The model under review builds one solid part; all positions refer to its coordinate system, in mm. A direction names the side the tool comes from. Round coordinates to 2 decimals unless told otherwise and drop trailing zeros. Loops run counter-clockwise (first coordinate to the right, second up) from the corner with the lowest first, then second, coordinate; pieces in that order, holes last. Notation, with made-up numbers: M -4.5,-8.75 L 52.5,-8.75 A18 cw 52.5,19.25 Z; hole C 87,-15 d11. An arc over 180 degrees is marked long. One line per question, with ' | ' between items.
from build123d import *

# Parameters (mm, degrees)
SKETCH1_R           = 50
BOSS_EXTRUDE1_DEPTH = 5
SKETCH2_R           = 7
BOSS_EXTRUDE2_DEPTH = 2
CUT_EXTRUDE1_REACH  = 7
SKETCH3_R           = 1.55


with BuildPart() as part:
    # Sketch1 → Boss-Extrude1 (new body)
    with BuildSketch(Plane.XY):
        Circle(SKETCH1_R)
        with BuildLine():
            ThreePointArc((-31.028947368, -9.767518887), (-28.10136985, -6.783592054), (-26.375, -2.976470225))
            Line((-26.375, -2.976470225), (-26.375, 2.976470225))
            ThreePointArc((-26.375, 2.976470225), (-28.10136985, 6.783592054), (-31.028947368, 9.767518887))
            ThreePointArc((-31.028947368, 9.767518887), (-34.223647748, 14.6974406), (-33.189728353, 20.480281537))
            ThreePointArc((-33.189728353, 20.480281537), (-27.577164466, 27.577164466), (-20.480281537, 33.189728353))
            ThreePointArc((-20.480281537, 33.189728353), (-14.6974406, 34.223647748), (-9.767518887, 31.028947368))
            ThreePointArc((-9.767518887, 31.028947368), (0, 26), (9.767518887, 31.028947368))
            ThreePointArc((9.767518887, 31.028947368), (14.6974406, 34.223647748), (20.480281537, 33.189728353))
            ThreePointArc((20.480281537, 33.189728353), (27.577164466, 27.577164466), (33.189728353, 20.480281537))
            ThreePointArc((33.189728353, 20.480281537), (34.223647748, 14.6974406), (31.028947368, 9.767518887))
            ThreePointArc((31.028947368, 9.767518887), (28.10136985, 6.783592054), (26.375, 2.976470225))
            Line((26.375, 2.976470225), (26.375, -2.976470225))
            ThreePointArc((26.375, -2.976470225), (28.10136985, -6.783592054), (31.028947368, -9.767518887))
            ThreePointArc((31.028947368, -9.767518887), (34.223647748, -14.6974406), (33.189728353, -20.480281537))
            ThreePointArc((33.189728353, -20.480281537), (27.577164466, -27.577164466), (20.480281537, -33.189728353))
            ThreePointArc((20.480281537, -33.189728353), (14.6974406, -34.223647748), (9.767518887, -31.028947368))
            ThreePointArc((9.767518887, -31.028947368), (0, -26), (-9.767518887, -31.028947368))
            ThreePointArc((-9.767518887, -31.028947368), (-14.6974406, -34.223647748), (-20.480281537, -33.189728353))
            ThreePointArc((-20.480281537, -33.189728353), (-27.577164466, -27.577164466), (-33.189728353, -20.480281537))
            ThreePointArc((-33.189728353, -20.480281537), (-34.223647748, -14.6974406), (-31.028947368, -9.767518887))
        make_face(mode=Mode.SUBTRACT)
    extrude(amount=BOSS_EXTRUDE1_DEPTH)

    # Sketch2 → Boss-Extrude2 (add)
    with BuildSketch(Plane.XY.offset(5)):
        with Locations((-38, 0)):
            Circle(SKETCH2_R)
        with Locations((0, 38)):
            Circle(SKETCH2_R)
        with Locations((38, 0)):
            Circle(SKETCH2_R)
        with Locations((0, -38)):
            Circle(SKETCH2_R)
    extrude(amount=BOSS_EXTRUDE2_DEPTH)

    # Sketch3 → Cut-Extrude1 (cut, up to next)
    with BuildSketch(Plane.XY.offset(5), mode=Mode.PRIVATE) as cut_extrude1_sk1:
        with Locations((-12.727922061, 38.183766184)):
            Circle(SKETCH3_R)
    cut_extrude1_tool1 = extrude(cut_extrude1_sk1.sketch, amount=-CUT_EXTRUDE1_REACH, mode=Mode.PRIVATE) & part.part
    add(cut_extrude1_tool1.solids().sort_by_distance((-12.727922, 38.183766, 5))[0], mode=Mode.SUBTRACT)
    # Sketch3 → Cut-Extrude1 (cut, up to next)
    with BuildSketch(Plane.XY.offset(5), mode=Mode.PRIVATE) as cut_extrude1_sk2:
        with Locations((38.183766184, 12.727922061)):
            Circle(SKETCH3_R)
    cut_extrude1_tool2 = extrude(cut_extrude1_sk2.sketch, amount=-CUT_EXTRUDE1_REACH, mode=Mode.PRIVATE) & part.part
    add(cut_extrude1_tool2.solids().sort_by_distance((38.183766, 12.727922, 5))[0], mode=Mode.SUBTRACT)
    # Sketch3 → Cut-Extrude1 (cut, up to next)
    with BuildSketch(Plane.XY.offset(5), mode=Mode.PRIVATE) as cut_extrude1_sk3:
        with Locations((12.727922061, -38.183766184)):
            Circle(SKETCH3_R)
    cut_extrude1_tool3 = extrude(cut_extrude1_sk3.sketch, amount=-CUT_EXTRUDE1_REACH, mode=Mode.PRIVATE) & part.part
    add(cut_extrude1_tool3.solids().sort_by_distance((12.727922, -38.183766, 5))[0], mode=Mode.SUBTRACT)
    # Sketch3 → Cut-Extrude1 (cut, up to next)
    with BuildSketch(Plane.XY.offset(5), mode=Mode.PRIVATE) as cut_extrude1_sk4:
        with Locations((-38.183766184, -12.727922061)):
            Circle(SKETCH3_R)
    cut_extrude1_tool4 = extrude(cut_extrude1_sk4.sketch, amount=-CUT_EXTRUDE1_REACH, mode=Mode.PRIVATE) & part.part
    add(cut_extrude1_tool4.solids().sort_by_distance((-38.183766, -12.727922, 5))[0], mode=Mode.SUBTRACT)
    # Sketch3 → Cut-Extrude1 (cut, up to next)
    with BuildSketch(Plane.XY.offset(5), mode=Mode.PRIVATE) as cut_extrude1_sk5:
        with Locations((-38.183766184, 12.727922061)):
            Circle(SKETCH3_R)
    cut_extrude1_tool5 = extrude(cut_extrude1_sk5.sketch, amount=-CUT_EXTRUDE1_REACH, mode=Mode.PRIVATE) & part.part
    add(cut_extrude1_tool5.solids().sort_by_distance((-38.183766, 12.727922, 5))[0], mode=Mode.SUBTRACT)
    # Sketch3 → Cut-Extrude1 (cut, up to next)
    with BuildSketch(Plane.XY.offset(5), mode=Mode.PRIVATE) as cut_extrude1_sk6:
        with Locations((12.727922061, 38.183766184)):
            Circle(SKETCH3_R)
    cut_extrude1_tool6 = extrude(cut_extrude1_sk6.sketch, amount=-CUT_EXTRUDE1_REACH, mode=Mode.PRIVATE) & part.part
    add(cut_extrude1_tool6.solids().sort_by_distance((12.727922, 38.183766, 5))[0], mode=Mode.SUBTRACT)
    # Sketch3 → Cut-Extrude1 (cut, up to next)
    with BuildSketch(Plane.XY.offset(5), mode=Mode.PRIVATE) as cut_extrude1_sk7:
        with Locations((38.183766184, -12.727922061)):
            Circle(SKETCH3_R)
    cut_extrude1_tool7 = extrude(cut_extrude1_sk7.sketch, amount=-CUT_EXTRUDE1_REACH, mode=Mode.PRIVATE) & part.part
    add(cut_extrude1_tool7.solids().sort_by_distance((38.183766, -12.727922, 5))[0], mode=Mode.SUBTRACT)
    # Sketch3 → Cut-Extrude1 (cut, up to next)
    with BuildSketch(Plane.XY.offset(5), mode=Mode.PRIVATE) as cut_extrude1_sk8:
        with Locations((-12.727922061, -38.183766184)):
            Circle(SKETCH3_R)
    cut_extrude1_tool8 = extrude(cut_extrude1_sk8.sketch, amount=-CUT_EXTRUDE1_REACH, mode=Mode.PRIVATE) & part.part
    add(cut_extrude1_tool8.solids().sort_by_distance((-12.727922, -38.183766, 5))[0], mode=Mode.SUBTRACT)


solid = part.part
1) Machinability: for faces 4 (the cylindrical face through (0, 26, 2)), 5 (the cylindrical face through (-0.91, -31.06, 5.99)), which of the approach directions +Z, -Z, +X, -X, +Y, -Y give a long, thin tool a straight path to every point of the face, cutting with its end or side? Answer none if there is none.
Output values:
face 4: +Z, -Z | face 5: +Z
2) Mouldability with a two-part tool opening along Y and no side actions: class faces 1 (the flat face through (0, 38, 7)), 2 (the cylindrical face through (44.677, 2.103, 5.986)), 3 (the cylindrical face through (14.615, 34.207, 2.465)) as +Y half, -Y half, draft (parallel to the pull), parting line (faces both ways), or undercut.
Output values:
face 1: draft | face 2: parting line | face 3: undercut
3) Add section C-C on x = -38. State the section outline as (y, z) points.
Output values:
outline: M -32.5,0 L -14.27,0 L -14.27,5 L -32.5,5 Z; M -11.19,0 L 11.19,0 L 11.19,5 L 7,5 L 7,7 L -7,7 L -7,5 L -11.19,5 Z; M 14.27,0 L 32.5,0 L 32.5,5 L 14.27,5 Z
4) For line 1 (Y direction, x = -28, z = 2.25); line 2 (X direction, y = -12.5, z = 3.25), list the stretches that pass through material, from the lowest coordinate up.
Output values:
line 1: y = -41.42 to -27.15, -6.63 to 6.63, 27.15 to 41.42 | line 2: x = -48.41 to -39.72, -36.65 to -33.43, 33.43 to 36.65, 39.72 to 48.41
5) Add section B-B on x = 0. State the section outline as (y, z) points, then the cut area to 3 significant figures.
Output values:
outline: M -50,0 L -26,0 L -26,5 L -31,5 L -31,7 L -45,7 L -45,5 L -50,5 Z; M 26,0 L 50,0 L 50,5 L 45,5 L 45,7 L 31,7 L 31,5 L 26,5 Z | area: 296 mm²
6) Insertion check: P1, Ø4, axis at x = 38.18, y = -12.73, coming from the +Z side; P2, Ø4, axis at x = -38.18, y = -12.73, coming from the -Z side; P3, Ø1.5, axis at y = 1, z = 2.5, coming from the +X side. Each pin has a flat end and moves straight along its axis. Give the tip position at first contact, or say it passes through.
Output values:
P1: stops at z = 5 | P2: stops at z = 0 | P3: stops at x = 50
7) Add section A-A on y = 0. State the section outline as (x, z) points (3 decimals), then the cut area to 3 significant figures.
Output values:
outline: M -50,0 L -26.375,0 L -26.375,5 L -31,5 L -31,7 L -45,7 L -45,5 L -50,5 Z; M 26.375,0 L 50,0 L 50,5 L 45,5 L 45,7 L 31,7 L 31,5 L 26.375,5 Z | area: 292 mm²
8) Add section D-D on x = 22. State the section outline as (y, z) points, then the cut area to 3 significant figures.
Output values:
outline: M -44.9,0 L -32.2,0 L -32.2,5 L -44.9,5 Z; M 32.2,0 L 44.9,0 L 44.9,5 L 32.2,5 Z | area: 127 mm²
